Source: CAD feature listing. Evaluate the final solid. Frame: model axes, mm. A direction names the side the tool comes from. Coordinates: 2 decimals unless noted, no trailing zeros. Loops run counter-clockwise (first coordinate to the right, second up) from the corner with the lowest first, then second, coordinate; pieces in that order, holes last. Notation, with made-up numbers: (-8, 86.5) -> (13, 86.5) arc R24 ccw to (13, 111.5) -> close; hole circle Ø2 at (-9.5, -10). An arc over 180 degrees is marked (long way). One line per question, with ' | ' between items. Start each with the question number.
```python
from build123d import *

# Parameters (mm, degrees)
SKETCH2_W          = 16.5
SKETCH2_H          = 15.5
SKETCH2_W_2        = 14.5
SKETCH2_H_2        = 3.4
CUT_EXTRUDE1_DEPTH = 2.3


with BuildPart() as part:
    # Sketch1 → Revolve1 (revolve)
    with BuildSketch(Plane.XY):
        Polygon((0, 7.05), (0, 3.175), (7.7, 3.175), (7.7, 7.25), (0.2, 7.25), align=None)
    revolve(axis=Axis((7.7, 0, 0), (-1, 0, 0)))

    # Sketch2 → Cut-Extrude1 (cut)
    with BuildSketch(Plane(origin=(7.7, 0, 0), x_dir=(0, 0, -1), z_dir=(1, 0, 0))):
        Rectangle(SKETCH2_W, SKETCH2_H)
        Rectangle(SKETCH2_W_2, SKETCH2_H_2, mode=Mode.SUBTRACT)
    extrude(amount=-CUT_EXTRUDE1_DEPTH, mode=Mode.SUBTRACT)

    # Sketch3 → Cut-Revolve1 (revolve, cut)
    with BuildSketch(Plane(origin=(2.6, 0, 0), x_dir=(0, 0, -1), z_dir=(1, 0, 0))):
        Polygon((-7.25, 0), (-7.25, 1.5), (-6.9795, 1.2295), (0, 1.2295), (0, 0), align=None)
    revolve(axis=Axis((2.6, 0, 0), (0, 0, 1)), mode=Mode.SUBTRACT)

    # Sketch4 → Cut-Revolve2 (revolve, cut)
    with BuildSketch(Plane(origin=(2.6, 0, 0), x_dir=(0, 0, -1), z_dir=(1, 0, 0))):
        Polygon((0, -7.25), (-1.5, -7.25), (-1.2295, -6.9795), (-1.2295, 0), (0, 0), align=None)
    revolve(axis=Axis((2.6, 0, 0), (0, -1, 0)), mode=Mode.SUBTRACT)


solid = part.part
```
(1) Ray query, L1, parallel to X at y = 0, z = 4; L2, parallel to Y at x = 4.25, z = 0 (3 decimals); L3, parallel to X at y = -5, z = 3.5. Return the intervals inside material, ascending.
(2) Contact query for flat-ended pins moving along their axis: pin 1 Ø7.5 at (y, z) = (0, 0) entering from +X; pin 2 Ø4 at (x, y) = (4, 5) entering from +Z; pin 3 Ø1.7 at (y, z) = (5.5, -2) entering from +X; pin 4 Ø4 at (x, y) = (4, -4) entering from +Z. Output: stop coordinate, or through.
(3) Access query for faces 5 (the cylindrical face through (3.064, 6.697, 2.777)), 6 (the cylindrical face through (2.231, -4.925, 1.173)), 7 (the flat face through (7, 1.7, 5)), 8 (the flat face through (5.4, -4, 0)), 9 (the flat face through (7.7, 0, -5)). Directions: +Z, -Z, +X, -X, +Y, -Y. A direction counts if a zero-diameter tool reaches every point of the face in a straight line with its end or side. Return the directions, or none.
(4) Draft query along Y for faces 1 (the cylindrical face through (2.231, 1.173, 4.925)), 2 (the cylindrical face through (3.05, 2.93, 1.22)), 3 (the flat face through (7, 1.7, -5)), 4 (the flat face through (5.4, 5, 0)). Return one class per face: pulls with the +Y half, pulls with the -Y half, needs draft (parallel to the pull), parting line crosses it, or undercut.
(5) Cut plane A-A, the plane z = 0. State how many separate pieces and enclosed holes the cut face has, and give its area (3 significant figures).
(6) Cut plane B-B, the plane x = 7. Return the cut outline in (y, z) (3 decimals), and give its area (3 significant figures).
Here are the results:
1) L1: x = 0 to 1.37, 3.83 to 7.7 | L2: y = -7.25 to -3.175, 3.175 to 7.25 | L3: x = 0 to 5.4
2) pin 1: stops at x = 7.7 | pin 2: stops at z = 6.6 | pin 3: stops at x = 5.4 | pin 4: stops at z = 6.97
3) face 5: +X, -X | face 6: -Y | face 7: +Z, -Z, +X, +Y | face 8: +Z, -Z, +X, -Y | face 9: +Z, -Z, +X, +Y, -Y
4) face 1: undercut | face 2: undercut | face 3: pulls with the +Y half | face 4: needs draft
5) separate pieces: 3 | enclosed holes: 0 | area: 33.9 mm2
6) outline: (-1.7, -7.048) arc R7.25 ccw to (1.7, -7.048) -> (1.7, -2.682) arc R3.175 cw to (-1.7, -2.682) -> close; (-1.7, 2.682) arc R3.175 cw to (1.7, 2.682) -> (1.7, 7.048) arc R7.25 ccw to (-1.7, 7.048) -> close | area: 28.3 mm2
